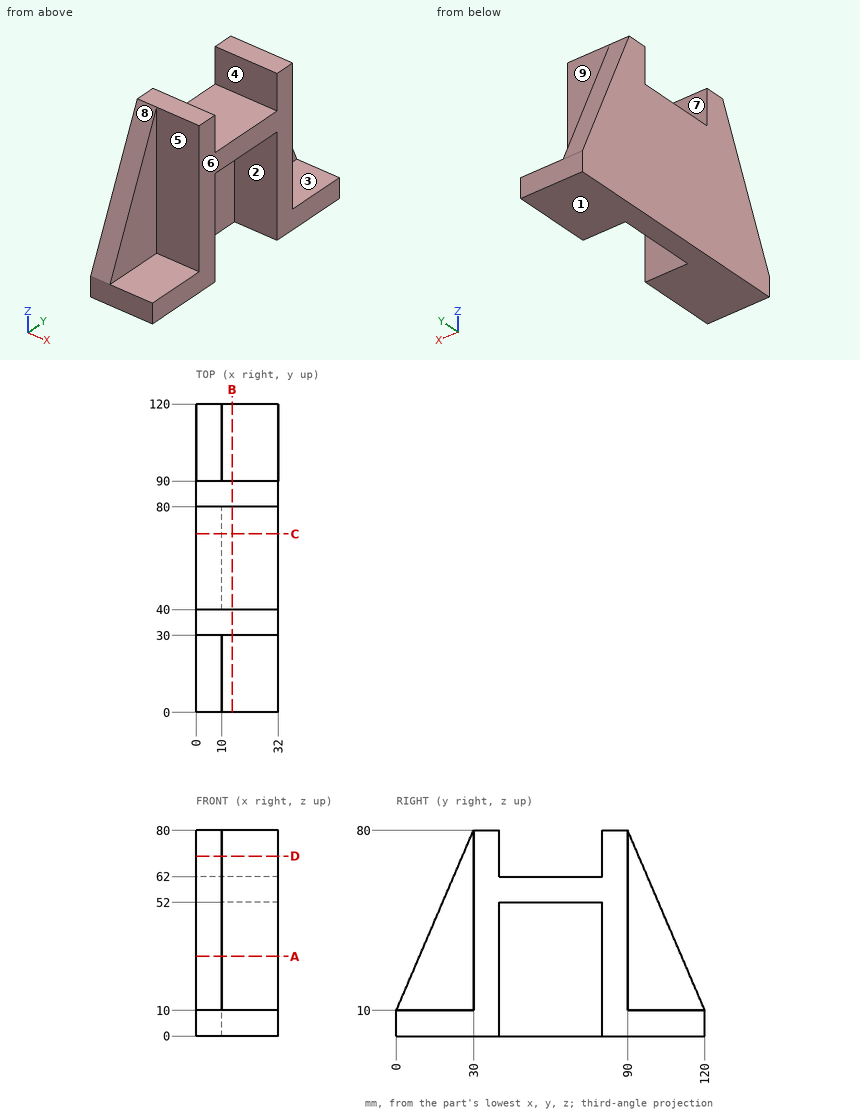
Geometry check sheet. Reference: drawing and pictorial views, mm from the part's lowest x, y, z. A direction names the side the tool comes from. Round coordinates to 2 decimals unless told otherwise and drop trailing zeros. Order: outer loops, then holes, each group sorted by start corner. A loop starts at its lowest first (then second) coordinate and runs counter-clockwise, first axis right, second up. Notation, with made-up numbers: M 15,47 L 45,47 A23 cw 45,56 Z; hole C 52,-25.5 d5. An arc over 180 degrees is marked long. Answer as CSV lines item,"result".
1) Thickness scan on probe 1 along Y at (x, z) = (14.5, 46.5); probe 2 along Y at (x, z) = (26.5, 9); probe 3 along X at (y, z) = (12, 34.5). Record the ranges inside material, lowest first. Write a range as [from, to].
Entries:
probe 1,"[30, 40], [80, 90]"
probe 2,"[0, 40], [80, 120]"
probe 3,"[0, 10]"
2) Mould release check, pull along Y, two halves, no side actions. Record for the marked faces 6, 7, 8 and 9: +Y half, -Y half, draft (parallel to the pull), parting line (faces both ways), or undercut.
Entries:
face 6,"draft"
face 7,"undercut"
face 8,"-Y half"
face 9,"+Y half"
3) Sectioned sample at C-C on y = 69.5. Record the cut outline in (x, z).
Entries:
outline,"M 0,0 L 10,0 L 10,52 L 32,52 L 32,62 L 0,62 Z"
4) Sectioned sample at B-B on x = 14. Record the cut outline in (y, z), and give its area (3 significant figures).
Entries:
outline,"M 0,0 L 40,0 L 40,52 L 80,52 L 80,0 L 120,0 L 120,10 L 90,10 L 90,80 L 80,80 L 80,62 L 40,62 L 40,80 L 30,80 L 30,10 L 0,10 Z"
area,"2,600 mm2"
5) Sectioned sample at D-D on z = 70. Record the cut outline in (x, y), and give its area (3 significant figures).
Entries:
outline,"M 0,25.71 L 10,25.71 L 10,30 L 32,30 L 32,40 L 0,40 Z; M 0,80 L 32,80 L 32,90 L 10,90 L 10,94.29 L 0,94.29 Z"
area,"726 mm2"
6) Tool access check on the marked faces 1, 2, 3, 4 and 5. Record the directions out of +Z, -Z, +X, -X, +Y, -Y that give a thin tool (end or side, any length) a straight path to the whole face; none if there is none.
Entries:
face 1,"-Z, +X, -X, +Y, -Y"
face 2,"-Z, +X"
face 3,"+Z, +X, +Y"
face 4,"+Z, +X, -X"
face 5,"+Z, +X, -Y"
7) Sectioned sample at A-A on z = 31. Record the cut outline in (x, y).
Entries:
outline,"M 0,9 L 10,9 L 10,30 L 32,30 L 32,40 L 10,40 L 10,80 L 32,80 L 32,90 L 10,90 L 10,111 L 0,111 Z"
8) Gauge pin test, flat ends, axial feed: pin 1 Ø24 at (y, z) = (106, 28.5) entering from +X; pin 2 Ø5 at (x, z) = (15, 27) entering from -Y; pin 3 Ø11 at (x, y) = (17.5, 107) entering from +Z. Record the tip position at first contact, or that the pin passes through.
Entries:
pin 1,"x = 10"
pin 2,"y = 30"
pin 3,"z = 10"
